Input: part model. Units: mm. Frame: model coordinates. Round coordinates to 2 decimals unless told otherwise and drop trailing zeros. Order: outer loops, then holes, each group sorted by start corner. A loop starts at its lowest first (then second) coordinate and runs counter-clockwise, first axis right, second up. Notation, with made-up numbers: (-34, -9) -> (14, -9) arc R26 ccw to (14, 22) -> close; hole circle Ø5 at (-24, -10). An arc over 180 degrees is marked (long way). Answer as CSV lines item,"result". Start each with the question number.
1) Section query A-A, the plane x = 1.5. Output: boundary loops of the cut face in (y, z), and give its area (3 significant figures).
2) First-contact query: P1, Ø3.5, axis at y = 309, z = -309, coming from the +X side. Flat tip, straight axial feed; report the tip coordinate or a pass-through.
3) Line query: L1, parallel to Y at x = 0.65, z = -309; L2, parallel to Y at x = 1.2, z = -309; L3, parallel to Z at x = 1.15, y = 309. Output: solid intervals per line, ascending.
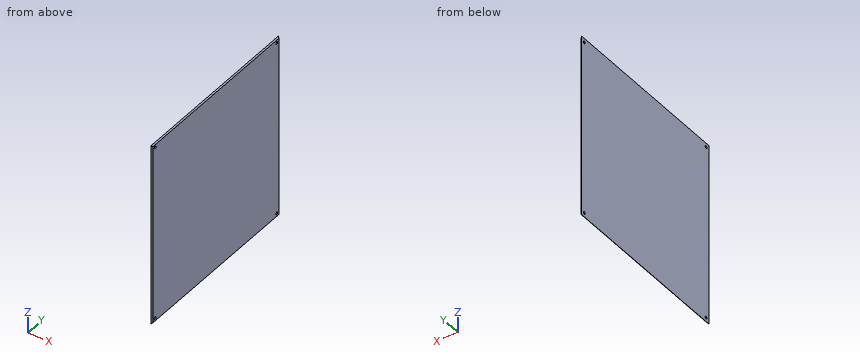
```python
from build123d import *

# Parameters (mm, degrees)
SKETCH1_W                = 316
SKETCH1_H                = 316
BOSS_EXTRUDE1_DEPTH      = 2
CHAMFER1_SIZE            = 2
M4_CLEARANCE_HOLE1_D     = 4.5
M4_CLEARANCE_HOLE1_DEPTH = 30
M4_CLEARANCE_HOLE1_TIP   = 1.351936393


with BuildPart() as part:
    # Sketch1 → Boss-Extrude1 (new body)
    with BuildSketch(Plane(origin=(0, 0, 0), x_dir=(0, 0, -1), z_dir=(1, 0, 0))):
        with Locations((158, 158)):
            Rectangle(SKETCH1_W, SKETCH1_H)
    extrude(amount=BOSS_EXTRUDE1_DEPTH)

    # Chamfer1
    chamfer1_edges = [part.edges().sort_by_distance(p)[0] for p in [
        (2, 158, 0),
        (2, 316, -158),
        (2, 158, -316),
        (2, 0, -158),
    ]]
    chamfer(chamfer1_edges, length=CHAMFER1_SIZE - 0.0001)  # a hair under: the kernel refuses the full size

    # M4 Clearance Hole1
    with Locations(Plane(origin=(2, 0, 0), x_dir=(0, 0, -1), z_dir=(1, 0, 0))):
        with Locations((7, 309), (309, 309), (309, 7), (7, 7)):
            Hole(M4_CLEARANCE_HOLE1_D / 2, depth=M4_CLEARANCE_HOLE1_DEPTH)
            with Locations((0, 0, -(M4_CLEARANCE_HOLE1_DEPTH + M4_CLEARANCE_HOLE1_TIP / 2))):  # 118° drill point
                Cone(0, M4_CLEARANCE_HOLE1_D / 2, M4_CLEARANCE_HOLE1_TIP, mode=Mode.SUBTRACT)


solid = part.part
```
Findings:
1,outline,"(1.5, -314.5) -> (314.5, -314.5) -> (314.5, -1.5) -> (1.5, -1.5) -> close; hole circle Ø4.5 at (7, -309); hole circle Ø4.5 at (7, -7); hole circle Ø4.5 at (309, -309); hole circle Ø4.5 at (309, -7)"
1,area,"97,900 mm^2"
2,P1,"passes through"
3,L1,"y = 0.65 to 4.75, 9.25 to 306.75, 311.25 to 315.35"
3,L2,"y = 1.2 to 4.75, 9.25 to 306.75, 311.25 to 314.8"
3,L3,"z = -314.85 to -311.25, -306.75 to -9.25, -4.75 to -1.15"
